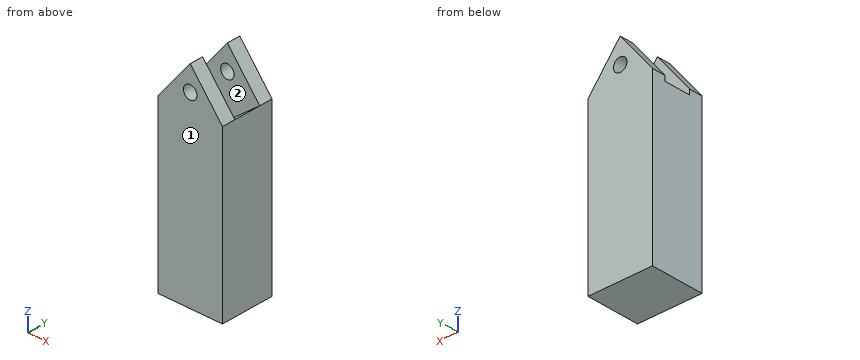
from build123d import *

# Parameters (mm, degrees)
F0_R     = 3.175
F1_DEPTH = 25.4
F2_W     = 12.7
F2_H     = 24.5806615153
F3_DEPTH = 25.4


with BuildPart() as f1:
    # F0 (on Front) → F1 (new body)
    with BuildSketch(Plane.XZ):
        Polygon((-20.1742626747, 33.7985328736), (-35.4142626747, 53.0845723978), (-50.6542626747, 33.7985328736), (-50.6542626747, -46.0891589454), (-20.1742626747, -46.0891589454), align=None)
        with Locations((-35.4142626747, 41.4804334976)):
            Circle(F0_R, mode=Mode.SUBTRACT)
    extrude(amount=F1_DEPTH)

    # F2 (on face) → F3 (cut)
    with BuildSketch(Plane(origin=(4.0221113088, 0, 3.1783081368), x_dir=(0, 1, 0), z_dir=(0.7846021358, 0, 0.6199995875))):
        with Locations((-12.7, 51.3167663736)):
            Rectangle(F2_W, F2_H)
    extrude(amount=-F3_DEPTH, mode=Mode.SUBTRACT)


solid = f1.part
For this review, take the finished solid that the model builds, in its own axes (mm). Face numbers are marked on the shaded views. A direction names the side the tool comes from. Coordinates: 2 decimals unless noted, no trailing zeros. Loops run counter-clockwise (first coordinate to the right, second up) from the corner with the lowest first, then second, coordinate; pieces in that order, holes last. Notation, with made-up numbers: (-16, 49) -> (-7, 49) arc R12 ccw to (-7, 54) -> close; hole circle Ø6 at (69.5, -26.5). An arc over 180 degrees is marked (long way). Write each question's results on one line, items separated by ' | '.
Q1. Machinability: for the marked faces 1 and 2, which of the approach directions +Z, -Z, +X, -X, +Y, -Y give a long, thin tool a straight path to every point of the face, cutting with its end or side? Answer none if there is none.
Taken from the geometry:
face 1: +Z, -Z, +X, -X, -Y | face 2: +Z
Q2. Add section B-B, the plane z = 25.5. State the section outline as (x, y) points.
Taken from the geometry:
outline: (-50.65, -25.4) -> (-20.17, -25.4) -> (-20.17, 0) -> (-50.65, 0) -> close; hole (-45.99, -19.05) -> (-30.68, -19.05) -> (-30.68, -6.35) -> (-45.99, -6.35) -> close
Q3. To check wall thickness, follow line 1 along Y through (x, z) = (-35.5, 31); line 2 along Z through (x, y) = (-25.5, -11); line 3 along Z through (x, y) = (-41, -8.25). State the ranges of each line that lie inside material, in increasing order. Write a range as [from, to].
Taken from the geometry:
line 1: [-25.4, -19.05], [-6.35, 0] | line 2: [-46.09, 29.59] | line 3: [-46.09, 19.19]
Q4. Add section A-A, the plane y = -7.75. State the section outline as (x, z) points.
Taken from the geometry:
outline: (-50.65, -46.09) -> (-20.17, -46.09) -> (-20.17, 33.8) -> (-40.1, 18.05) -> (-50.65, 31.4) -> close
Q5. Add section C-C, the plane x = -42. State the section outline as (y, z) points.
Taken from the geometry:
outline: (-25.4, -46.09) -> (0, -46.09) -> (0, 44.75) -> (-6.35, 44.75) -> (-6.35, 20.45) -> (-19.05, 20.45) -> (-19.05, 44.75) -> (-25.4, 44.75) -> close
Q6. Add section D-D, the plane y = -2.5. State the section outline as (x, z) points (3 decimals), then the cut area to 3 significant figures.
Taken from the geometry:
outline: (-50.654, -46.089) -> (-20.174, -46.089) -> (-20.174, 33.799) -> (-35.414, 53.085) -> (-50.654, 33.799) -> close; hole circle Ø6.35 at (-35.414, 41.48) | area: 2,700 mm²
Q7. For pin 1 Ø1.5 at (y, z) = (-21, 39) entering from +X; pin 2 Ø5 at (x, y) = (-30.5, -3.5) entering from +Z, all flat-tipped, find the tip position at first contact; note any pin that passes through.
Taken from the geometry:
pin 1: x = -23.69 | pin 2: z = 50.03
